CAD build for the part. Positions are in the model's coordinates, mm. Round coordinates to 2 decimals unless told otherwise and drop trailing zeros. Loops run counter-clockwise (first coordinate to the right, second up) from the corner with the lowest first, then second, coordinate; pieces in that order, holes last. Notation, with made-up numbers: M 35.25,50.25 L 82.25,50.25 A11 cw 82.25,60.25 Z; hole C 9.5,-22 d11. An arc over 180 degrees is marked long. Put each result on its own line as item: value. Start each with the question number.
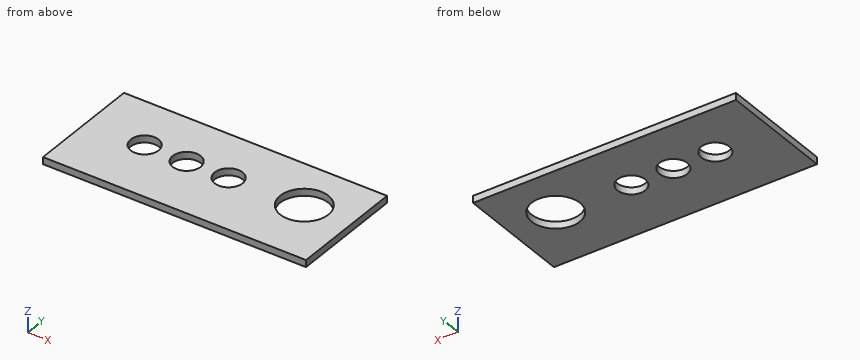
from build123d import *

# Parameters (mm, degrees)
MODEL_W             = 477.189260789
MODEL_H             = 209.095023119
BOSS_EXTRUDE1_DEPTH = 12.7


with BuildPart() as part:
    # Model → Boss-Extrude1 (new body)
    with BuildSketch(Plane.XY):
        with Locations((245.803972347, 112.449415536)):
            Rectangle(MODEL_W, MODEL_H)
        with BuildLine():
            ThreePointArc((239.098491904, 121.096908294), (264.498491904, 95.696908294), (289.898491904, 121.096908294))
            ThreePointArc((289.898491904, 121.096908294), (264.498491904, 146.496908294), (239.098491904, 121.096908294))
        make_face(mode=Mode.SUBTRACT)
        with BuildLine():
            ThreePointArc((162.898491904, 121.096908294), (188.298491904, 95.696908294), (213.698491904, 121.096908294))
            ThreePointArc((213.698491904, 121.096908294), (188.298491904, 146.496908294), (162.898491904, 121.096908294))
        make_face(mode=Mode.SUBTRACT)
        with BuildLine():
            ThreePointArc((137.498491904, 121.096908294), (112.098491904, 146.496908294), (86.698491904, 121.096908294))
            ThreePointArc((86.698491904, 121.096908294), (112.098491904, 95.696908294), (137.498491904, 121.096908294))
        make_face(mode=Mode.SUBTRACT)
        with BuildLine():
            ThreePointArc((442.018972347, 126.103389526), (398.203972347, 169.918389526), (354.388972347, 126.103389526))
            ThreePointArc((354.388972347, 126.103389526), (398.203972347, 82.288389526), (442.018972347, 126.103389526))
        make_face(mode=Mode.SUBTRACT)
    extrude(amount=BOSS_EXTRUDE1_DEPTH)


solid = part.part
(1) Cut at A-A on x = 373. List the corners of the cut face in (y, z).
(2) Drill centre lines: line 1 along X through (y, z) = (119.5, 12); line 2 along X through (y, z) = (131.5, 2.25); line 3 along X through (y, z) = (151.5, 8.25). Where is each one in solid material? Low to high.
(3) Cut at C-C on z = 9.75. List the corners of the cut face in (x, y) (1 decimal).
(4) Cut at D-D on y = 135. List the corners of the cut face in (x, z).
(5) Cut at B-B on y = 89. List the corners of the cut face in (x, z), and give its area (3 significant figures).
Taken from the geometry:
1. outline: M 7.9,0 L 90.26,0 L 90.26,12.7 L 7.9,12.7 Z; M 161.94,0 L 217,0 L 217,12.7 L 161.94,12.7 Z
2. line 1: 7.21 to 86.75, 137.45 to 162.95, 213.65 to 239.15, 289.85 to 354.89, 441.52 to 484.4
2. line 2: 7.21 to 88.93, 135.27 to 165.13, 211.47 to 241.33, 287.67 to 354.72, 441.69 to 484.4
2. line 3: 7.21 to 362.5, 433.91 to 484.4
3. outline: M 7.2,7.9 L 484.4,7.9 L 484.4,217 L 7.2,217 Z; hole C 112.1,121.1 d50.8; hole C 188.3,121.1 d50.8; hole C 264.5,121.1 d50.8; hole C 398.2,126.1 d87.6
4. outline: M 7.21,0 L 90.84,0 L 90.84,12.7 L 7.21,12.7 Z; M 133.36,0 L 167.04,0 L 167.04,12.7 L 133.36,12.7 Z; M 209.56,0 L 243.24,0 L 243.24,12.7 L 209.56,12.7 Z; M 285.76,0 L 355.3,0 L 355.3,12.7 L 285.76,12.7 Z; M 441.11,0 L 484.4,0 L 484.4,12.7 L 441.11,12.7 Z
5. outline: M 7.21,0 L 374.9,0 L 374.9,12.7 L 7.21,12.7 Z; M 421.51,0 L 484.4,0 L 484.4,12.7 L 421.51,12.7 Z
5. area: 5,470 mm2
